```python
from build123d import *

# Parameters (mm, degrees)
SKETCH1_W                    = 10
SKETCH1_H                    = 3
BOSS_EXTRUDE1_DEPTH          = 3
F_90_0_0087_DIAMETER_HOLE1_D = 0.22098
SKETCH15_W                   = 3
SKETCH15_H                   = 3
BOSS_EXTRUDE2_DEPTH          = 7
M2X0_4_TAPPED_HOLE1_D        = 1.6
M2X0_4_TAPPED_HOLE1_DEPTH    = 5
M2X0_4_TAPPED_HOLE1_TIP      = 0.480688495
FILLET4_R                    = 0.5
FILLET3_R                    = 1.5


with BuildPart() as part:
    # Sketch1 → Boss-Extrude1 (new body)
    with BuildSketch(Plane(origin=(0, 0, 0), x_dir=(1, 0, 0), z_dir=(0, 1, 0))):
        Rectangle(SKETCH1_W, SKETCH1_H)
    extrude(amount=BOSS_EXTRUDE1_DEPTH)

    # 90 _0.0087_ Diameter Hole1 (through all)
    with Locations(Plane(origin=(0, 3, 0), x_dir=(1, 0, 0), z_dir=(0, 1, 0))):
        with Locations((0.5, 0), (-0.5, 0)):
            Hole(F_90_0_0087_DIAMETER_HOLE1_D / 2)

    # Sketch8 → Tap Drill for M2x0.4 Tap1 (revolve, cut)
    with BuildSketch(Plane(origin=(-5, 1.5, 0), x_dir=(0, 0, 1), z_dir=(0, 1, 0))):
        Polygon((0, 0), (0, 4.85), (0.8, 4.369311505), (0.8, 0), align=None)
    tap_drill_for_m2x0_4_tap1 = revolve(axis=Axis((-11.35, 1.5, 0), (1, 0, 0)), mode=Mode.SUBTRACT)

    # Mirror1: Tap Drill for M2x0.4 Tap1 across plane
    add(tap_drill_for_m2x0_4_tap1.mirror(Plane(origin=(0, 0, 0), x_dir=(0, 0, 1), z_dir=(1, 0, 0))), mode=Mode.SUBTRACT)

    # Sketch15 → Boss-Extrude2 (add)
    with BuildSketch(Plane.XY.offset(1.5)):
        with Locations((0, 1.5)):
            Rectangle(SKETCH15_W, SKETCH15_H)
    extrude(amount=BOSS_EXTRUDE2_DEPTH)

    # M2x0.4 Tapped Hole1
    with Locations(Plane.XY.offset(8.5)):
        with Locations((0, 1.5)):
            Hole(M2X0_4_TAPPED_HOLE1_D / 2, depth=M2X0_4_TAPPED_HOLE1_DEPTH)
            with Locations((0, 0, -(M2X0_4_TAPPED_HOLE1_DEPTH + M2X0_4_TAPPED_HOLE1_TIP / 2))):  # 118° drill point
                Cone(0, M2X0_4_TAPPED_HOLE1_D / 2, M2X0_4_TAPPED_HOLE1_TIP, mode=Mode.SUBTRACT)

    # Fillet4
    fillet4_edges = [part.edges().sort_by_distance(p)[0] for p in [
        (-3.25, 3, 1.5),
        (3.25, 0, 1.5),
        (3.25, 3, 1.5),
        (-3.25, 0, 1.5),
        (0, 0, -1.5),
        (0, 3, -1.5),
    ]]
    fillet(fillet4_edges, radius=FILLET4_R)

    # Fillet3
    # the kernel refuses this fillet: 1.5 mm, written as the material it adds along each edge
    with BuildSketch(Plane(origin=(1.5, 0.5, 1.5), x_dir=(1, 0, 0), z_dir=(0, 1, 0)), Plane(origin=(-1.5, 2.5, 1.5), x_dir=(-1, 0, 0), z_dir=(0, -1, 0))) as fillet3_piece_1:
        with BuildLine():
            CenterArc((FILLET3_R, -FILLET3_R), FILLET3_R, 90, 90)
            Line((0, -FILLET3_R), (0, 0))
            Line((0, 0), (FILLET3_R, 0))
        make_face()
    extrude(amount=2)
    with BuildSketch(Plane(origin=(1.5, 0.5, 1), x_dir=(0, 0.006283143965558625, 0.9999802608561371), z_dir=(0, -0.9999802608561371, 0.006283143965558625))) as fillet3_piece_2_section:
        with BuildLine():
            CenterArc((-0.5 - FILLET3_R, -FILLET3_R), FILLET3_R, 0, 90)
            Line((-0.5 - FILLET3_R, 0), (-0.5, 0))
            Line((-0.5, 0), (-0.5, -FILLET3_R))
        make_face()
    fillet3_piece_2 = revolve(axis=Axis((1.5, 0.5, 1), (-1, 0, 0)), revolution_arc=359.64, mode=Mode.PRIVATE)
    fillet3_piece_2 = fillet3_piece_2 - Plane(origin=(2.067816643, 1.5, 0), x_dir=(0, 0, 1), z_dir=(1, 0, 0)) * Cylinder(0.8, 8, mode=Mode.PRIVATE)
    fillet3_piece_2 = split(fillet3_piece_2, bisect_by=Plane(origin=(2.067816643, 0, 1.382028407), z_dir=(0, 1, 0)), keep=Keep.TOP, mode=Mode.PRIVATE)
    add(fillet3_piece_2)
    with BuildSketch(Plane(origin=(1.5, 2.5, 1), x_dir=(0, -0.006283143965558403, 0.9999802608561371), z_dir=(0, 0.9999802608561371, 0.006283143965558403))) as fillet3_piece_3_section:
        with BuildLine():
            CenterArc((-0.5 - FILLET3_R, FILLET3_R), FILLET3_R, 270, 90)
            Line((-0.5 - FILLET3_R, 0), (-0.5, 0))
            Line((-0.5, 0), (-0.5, FILLET3_R))
        make_face()
    fillet3_piece_3 = revolve(axis=Axis((1.5, 2.5, 1), (1, 0, 0)), revolution_arc=359.64, mode=Mode.PRIVATE)
    fillet3_piece_3 = split(fillet3_piece_3, bisect_by=Plane(origin=(2.067816643, 3, 1.382028407), z_dir=(0, -1, 0)), keep=Keep.TOP, mode=Mode.PRIVATE)
    fillet3_piece_3 = fillet3_piece_3 - Plane(origin=(2.067816643, 1.5, 0), x_dir=(0, 0, 1), z_dir=(1, 0, 0)) * Cylinder(0.8, 8, mode=Mode.PRIVATE)
    add(fillet3_piece_3)
    with BuildSketch(Plane(origin=(-1.5, 0.5, 1), x_dir=(0, 0, 1), z_dir=(0, 1, 0))) as fillet3_piece_4_section:
        with BuildLine():
            CenterArc((0.5 + FILLET3_R, -FILLET3_R), FILLET3_R, 90, 90)
            Line((0.5 + FILLET3_R, 0), (0.5, 0))
            Line((0.5, 0), (0.5, -FILLET3_R))
        make_face()
    fillet3_piece_4 = revolve(axis=Axis((-1.5, 0.5, 1), (1, 0, 0)), revolution_arc=359.64, mode=Mode.PRIVATE)
    fillet3_piece_4 = fillet3_piece_4 - Plane(origin=(-2.067816642, 1.5, 0), x_dir=(0, 0, 1), z_dir=(-1, 0, 0)) * Cylinder(0.8, 8, mode=Mode.PRIVATE)
    fillet3_piece_4 = split(fillet3_piece_4, bisect_by=Plane(origin=(-2.067816642, 0, 1.382028407), z_dir=(0, 1, 0)), keep=Keep.TOP, mode=Mode.PRIVATE)
    add(fillet3_piece_4)
    with BuildSketch(Plane(origin=(-1.5, 2.5, 1), x_dir=(0, 0, 1), z_dir=(0, -1, 0))) as fillet3_piece_5_section:
        with BuildLine():
            CenterArc((0.5 + FILLET3_R, FILLET3_R), FILLET3_R, 180, 90)
            Line((0.5 + FILLET3_R, 0), (0.5, 0))
            Line((0.5, 0), (0.5, FILLET3_R))
        make_face()
    fillet3_piece_5 = revolve(axis=Axis((-1.5, 2.5, 1), (-1, 0, 0)), revolution_arc=359.64, mode=Mode.PRIVATE)
    fillet3_piece_5 = fillet3_piece_5 - Plane(origin=(-2.067816642, 1.5, 0), x_dir=(0, 0, 1), z_dir=(-1, 0, 0)) * Cylinder(0.8, 8, mode=Mode.PRIVATE)
    fillet3_piece_5 = split(fillet3_piece_5, bisect_by=Plane(origin=(-2.067816642, 3, 1.382028407), z_dir=(0, -1, 0)), keep=Keep.TOP, mode=Mode.PRIVATE)
    add(fillet3_piece_5)


solid = part.part
```
Geometry check sheet. Reference: the model listing, model coordinates, mm. A direction names the side the tool comes from. Round coordinates to 2 decimals unless told otherwise and drop trailing zeros. Order: outer loops, then holes, each group sorted by start corner. A loop starts at its lowest first (then second) coordinate and runs counter-clockwise, first axis right, second up. Notation, with made-up numbers: M 5.25,76.5 L 60.25,76.5 A25 ccw 60.25,97.5 Z; hole C -19.5,49 d2. An arc over 180 degrees is marked long. Write item = value, one per line.
Q1. Scan lines: line 1 (X direction, y = 0.8, z = 5.5); line 2 (Y direction, x = -2.3, z = 0); line 3 (Z direction, x = -3.2, y = 1.5). Record each from-to range of solid material in increasing order.
Answer block:
line_1 = -1.5 to -0.39, 0.39 to 1.5
line_2 = 0 to 0.7, 2.3 to 3
line_3 = -1.5 to -0.8, 0.8 to 1.5
Q2. Section check A-A (x = -4.25). Enter the section's corners in (y, z), plus the area to 3 significant figures.
Answer block:
outline = M 0,-1 A0.5 ccw 0.5,-1.5 L 2.5,-1.5 A0.5 ccw 3,-1 L 3,1 A0.5 ccw 2.5,1.5 L 0.5,1.5 A0.5 ccw 0,1 Z; hole C 1.5,0 d1.6
area = 6.77 mm^2
Q3. Depth check by flat-ended pin: pin 1 Ø1.3 at (y, z) = (1.5, 0) entering from +X; pin 2 Ø1.5 at (y, z) = (2, 6.5) entering from -X; pin 3 Ø0.9 at (y, z) = (2, 6) entering from +X. Enter the tip coordinate at first touch or a pass-through.
Answer block:
pin_1 = 0.54
pin_2 = -1.5
pin_3 = 1.5
Q4. Section check B-B (z = 3.75). Enter the section's corners in (x, y), plus the area to 3 significant figures.
Answer block:
outline = M -1.5,0 L 1.5,0 L 1.5,3 L -1.5,3 Z; hole C 0,1.5 d1.6
area = 6.99 mm^2
Q5. Section check C-C (y = 0.25). Give the number of separate pieces and of enclosed holes in the cut face, plus the area to 3 significant figures.
Answer block:
separate_pieces = 1
enclosed_holes = 2
area = 50.8 mm^2
Q6. Release check for a two-part mould opening along Z. For faces 4 (the flat face through (4, 1, 1.5)), 5 (the cylindrical face through (-2.85, 2.28, -0.17)), 6 (the cylindrical face through (2.85, 2.28, -0.17)), 7 (the flat face through (0, 3, 3)) record: released by +Z, released by -Z, zero draft, split by the parting line, or undercut.
Answer block:
face_4 = released by +Z
face_5 = undercut
face_6 = undercut
face_7 = zero draft
Q7. Set-up check for faces 1 (the flat face through (-4, 1, 1.5)), 2 (the cylindrical face through (0.17, 0.72, 5.96)), 3 (the flat face through (1.5, 1, 6)): record each of +Z, -Z, +X, -X, +Y, -Y from which the full face is reachable in a straight line by a thin tool's end or side.
Answer block:
face_1 = +Z, -X, +Y, -Y
face_2 = +Z
face_3 = +Z, +X, +Y, -Y
